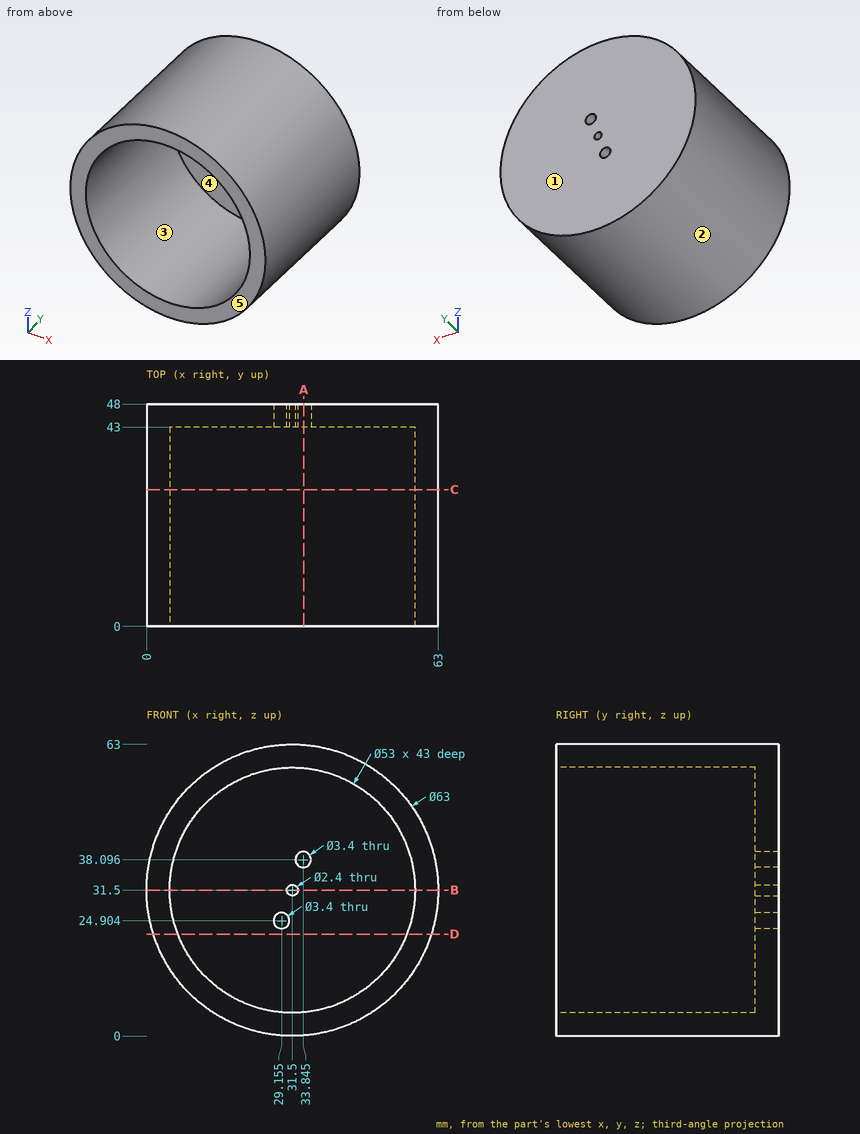
Geometry: see drawing. Coordinates: mm, zero at the bounding-box minimum. A direction names the side the tool comes from. Give positions to 0.01 mm unless a question says otherwise; leave off trailing zeros. Loops run counter-clockwise (first coordinate to the right, second up) from the corner with the lowest first, then second, coordinate; pieces in that order, holes last. Notation, with made-up numbers: (34, 5) - (51, 5) arc R17 ccw to (51, 20) - close; hole circle Ø2 at (-19, 6). An arc over 180 degrees is marked (long way). Use CSV: the item, a comma, the result in double quotes. Start each with the question number.
1. Section A-A (x = 34). Output: boundary loops of the cut face in (y, z).
2. Section C-C (y = 29.5). Output: boundary loops of the cut face in (x, z), then the cut area to 3 significant figures.
3. Reachability of the marked faces 4 and 5 from +Z, -Z, +X, -X, +Y, -Y: full face, straight path, thin tool, end or side. Return the list, or none.
4. Ray query, L1, parallel to X at y = 20, z = 31.5; L2, parallel to Z at x = 31.5, y = 44.2; L3, parallel to X at y = 31.5, z = 53.5 (1 decimal). Return the intervals inside material, ascending.
5. Draft query along Z for the marked faces 1, 2 and 3. Return one class per face: +Z half, -Z half, draft (parallel to the pull), parting line (faces both ways), or undercut.
6. Section D-D (z = 22). Output: boundary loops of the cut face in (x, y).
7. Pin query (flat end, axial travel): pin 1 (12 mm diameter, centred on y = 18.5, z = 52.5, fed in from -X); pin 2 (4 mm diameter, centred on x = 47, y = 41, fed in from -Z); pin 3 (1 mm diameter, centred on y = 9.5, z = 7.5, fed in from +X) (1 decimal). Return the tip coordinate at first contact, or that it passes through.
8. Section B-B (z = 31.5). Output: boundary loops of the cut face in (x, y).
Response:
1,outline,"(0, 0.1) - (48, 0.1) - (48, 36.4) - (43, 36.4) - (43, 5.12) - (0, 5.12) - close; (0, 57.88) - (43, 57.88) - (43, 39.79) - (48, 39.79) - (48, 62.9) - (0, 62.9) - close"
2,outline,"circle Ø63 at (31.5, 31.5); hole circle Ø53 at (31.5, 31.5)"
2,area,"911 mm²"
3,face 4,"-Y"
3,face 5,"+Z, -Z, +X, -X, -Y"
4,L1,"0 to 5, 58 to 63"
4,L2,"0 to 30.3, 32.7 to 63"
4,L3,"9 to 16.7, 46.3 to 54"
5,face 1,"draft"
5,face 2,"parting line"
5,face 3,"undercut"
6,outline,"(1.47, 0) - (6.76, 0) - (6.76, 43) - (56.24, 43) - (56.24, 0) - (61.53, 0) - (61.53, 48) - (1.47, 48) - close"
7,pin 1,"x = 3.8"
7,pin 2,"z = 3.04"
7,pin 3,"x = 52.5"
8,outline,"(0, 0) - (5, 0) - (5, 43) - (30.3, 43) - (30.3, 48) - (0, 48) - close; (32.7, 43) - (58, 43) - (58, 0) - (63, 0) - (63, 48) - (32.7, 48) - close"
